Could you check a few things on this drawing? It's one solid part, dimensions in mm from its lowest x, y, z. Coordinates: 2 decimals unless noted, no trailing zeros. Loops run counter-clockwise (first coordinate to the right, second up) from the corner with the lowest first, then second, coordinate; pieces in that order, holes last. Notation, with made-up numbers: M 1,60 L 33,60 A29 cw 33,92 Z; hole C 63,-10.5 d10. An arc over 180 degrees is marked long. Answer as a JSON object with one key per item and string values. Group by question number.
Item 1: Suppose I cut it at C-C (x = 65). Write out the boundary of the cut face in (y, z).
Item 2: Suppose I cut it at A-A (y = 15). Write out the boundary of the cut face in (x, z), then the cut area to 3 significant figures.
Item 3: If I drill on line 1 (X direction, y = 14.5, z = 12.75); line 2 (Y direction, x = 15, z = 5.5); line 3 (X direction, y = 8, z = 22), over which ranges is the centre line in solid material (lowest first)?
Item 4: We'd pull the mould along X, two halves only. Please class the marked faces 1, 2 and 3: +X half, -X half, draft (parallel to the pull), parting line (faces both ways), or undercut.
Item 5: I'm going to push flat-ended pins straight in: pin 1 Ø12 at (x, z) = (68.5, 11.5) entering from -Y; pin 2 Ø4 at (x, z) = (32.5, 10.5) entering from -Y; pin 3 Ø4 at (x, z) = (59, 22) entering from -Y; pin 4 Ø8 at (y, z) = (21, 14.5) entering from -X. Where does each tip first touch, or does it pass through?
Item 6: Suppose I cut it at B-B (z = 8.25). Write out the boundary of the cut face in (x, y), then the cut area to 3 significant figures.
Item 7: Suppose I cut it at D-D (x = 33.5). Write out the boundary of the cut face in (y, z).
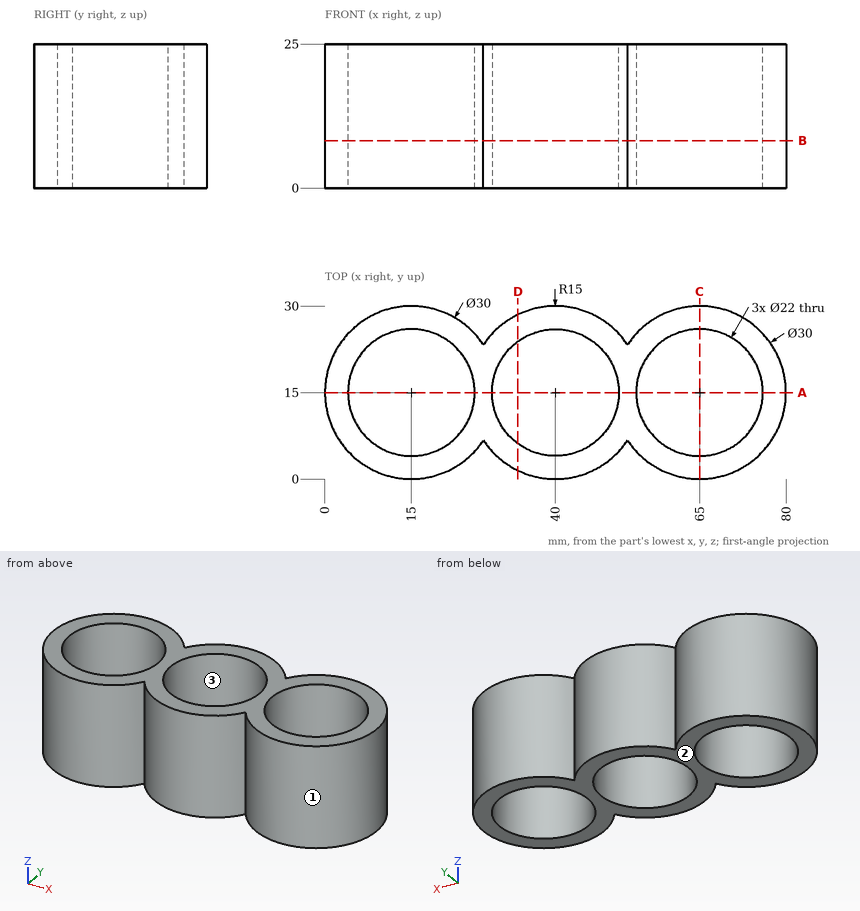
From the geometry:
{
 "1": {"outline": "M 0,0 L 4,0 L 4,25 L 0,25 Z; M 26,0 L 30,0 L 30,25 L 26,25 Z"},
 "2": {"outline": "M 0,0 L 4,0 L 4,25 L 0,25 Z; M 26,0 L 29,0 L 29,25 L 26,25 Z; M 51,0 L 54,0 L 54,25 L 51,25 Z; M 76,0 L 80,0 L 80,25 L 76,25 Z", "area": "350 mm2"},
 "3": {"line 1": "0.01 to 4.01, 25.99 to 29.01, 50.99 to 54.01, 75.99 to 79.99", "line 2": "0 to 4, 26 to 30", "line 3": "1.73 to 6.51, 23.49 to 31.51, 48.49 to 56.51, 73.49 to 78.27"},
 "4": {"face 1": "undercut", "face 2": "draft", "face 3": "undercut"},
 "5": {"pin 1": "y = 0", "pin 2": "y = 1.04", "pin 3": "y = 0.54", "pin 4": "x = 0.13"},
 "6": {"outline": "M 27.5,6.71 A15 ccw 52.5,6.71 A15 ccw long 52.5,23.29 A15 ccw 27.5,23.29 A15 ccw long Z; hole C 15,15 d22; hole C 40,15 d22; hole C 65,15 d22", "area": "868 mm2"},
 "7": {"outline": "M 1.48,0 L 6.13,0 L 6.13,25 L 1.48,25 Z; M 23.87,0 L 28.52,0 L 28.52,25 L 23.87,25 Z"}
}
